from build123d import *

# Parameters (mm, degrees)
SKETCH1_W           = 133.8
SKETCH1_H           = 16.37
SKETCH1_R           = 3.3
BOSS_EXTRUDE1_DEPTH = 1.38
SKETCH2_W           = 1.38
SKETCH2_H           = 16.37
BOSS_EXTRUDE2_DEPTH = 30
FILLET1_R           = 1.5
FILLET2_R           = 0.5
SKETCH3_R           = 2.6
CUT_EXTRUDE1_DEPTH  = 137.56


with BuildPart() as part:
    # Sketch1 → Boss-Extrude1 (new body)
    with BuildSketch(Plane(origin=(0, 0, 0), x_dir=(1, 0, 0), z_dir=(0, 1, 0))):
        with Locations((-5.141278074, 20.650419702)):
            Rectangle(SKETCH1_W, SKETCH1_H)
        with Locations((-30.141278074, 20.650419702)):
            Circle(SKETCH1_R, mode=Mode.SUBTRACT)
        with Locations((19.858721926, 20.650419702)):
            Circle(SKETCH1_R, mode=Mode.SUBTRACT)
    extrude(amount=BOSS_EXTRUDE1_DEPTH)

    # Sketch2 → Boss-Extrude2 (add)
    with BuildSketch(Plane(origin=(0, 1.38, 0), x_dir=(1, 0, 0), z_dir=(0, 1, 0))):
        with Locations((-72.731278074, 20.650419702)):
            Rectangle(SKETCH2_W, SKETCH2_H)
        with Locations((62.448721926, 20.650419702)):
            Rectangle(SKETCH2_W, SKETCH2_H)
    extrude(amount=-BOSS_EXTRUDE2_DEPTH)

    # Fillet1
    fillet1_edges = [part.edges().sort_by_distance(p)[0] for p in [
        (-73.421278074, 1.38, -20.650419702),
        (63.138721926, 1.38, -20.650419702),
    ]]
    fillet(fillet1_edges, radius=FILLET1_R)

    # Fillet2
    fillet2_edges = [part.edges().sort_by_distance(p)[0] for p in [
        (-72.041278074, 0, -20.650419702),
        (61.758721926, 0, -20.650419702),
    ]]
    fillet(fillet2_edges, radius=FILLET2_R)

    # Sketch3 → Cut-Extrude1 (cut, through all)
    with BuildSketch(Plane.ZY.offset(73.421278074)):
        with Locations((-20.650419702, -19.12)):
            Circle(SKETCH3_R)
    extrude(amount=-CUT_EXTRUDE1_DEPTH, mode=Mode.SUBTRACT)


solid = part.part
Input: part model. Units: mm. Frame: model coordinates. A direction names the side the tool comes from. Give positions to 0.01 mm unless a question says otherwise; leave off trailing zeros. Order: outer loops, then holes, each group sorted by start corner. A loop starts at its lowest first (then second) coordinate and runs counter-clockwise, first axis right, second up. Notation, with made-up numbers: (17.25, 3.5) -> (23.25, 3.5) arc R18 ccw to (23.25, 15.5) -> close; hole circle Ø1 at (-28, 83). An arc over 180 degrees is marked (long way). Use one line per item in the form item = value.
1) Section C-C, the plane y = -19.12. Return loops of the section in (x, z).
Response values:
outline = (-73.42, -28.84) -> (-72.04, -28.84) -> (-72.04, -23.25) -> (-73.42, -23.25) -> close; (-73.42, -18.05) -> (-72.04, -18.05) -> (-72.04, -12.47) -> (-73.42, -12.47) -> close; (61.76, -28.84) -> (63.14, -28.84) -> (63.14, -23.25) -> (61.76, -23.25) -> close; (61.76, -18.05) -> (63.14, -18.05) -> (63.14, -12.47) -> (61.76, -12.47) -> close
2) Reachability of faces 5 (the flat face through (61.759, -14, -21)), 6 (the cylindrical face through (19.429, 0.68, -23.922)) from +Z, -Z, +X, -X, +Y, -Y: full face, straight path, thin tool, end or side. Return the list, or none.
Response values:
face_5 = +Z, -Z, -Y
face_6 = +Y, -Y
3) First-contact query: pin 1 Ø5 at (x, z) = (12.5, -21.5) entering from -Y; pin 2 Ø5.5 at (x, z) = (-30.14, -20.65) entering from -Y. Flat tips, straight axial feed; report the tip coordinate or a pass-through.
Response values:
pin_1 = 0
pin_2 = through
4) Line query: probe 1 along X at (y, z) = (-21.25, -27.25); probe 2 along Y at (x, z) = (-52, -14.5). Output: solid intervals per line, ascending.
Response values:
probe_1 = -73.42 to -72.04, 61.76 to 63.14
probe_2 = 0 to 1.38
5) Mould query, pull axis Y, two halves, no side actions, for faces 1 (the cylindrical face through (62.44, -19.01, -23.25)), 2 (the cylindrical face through (-72.74, -19.01, -23.25)), 3 (the flat face through (-6, 1.38, -21)), 4 (the flat face through (-5, 1, -28.835)). Classes: pulls with the +Y half, pulls with the -Y half, needs draft (parallel to the pull), parting line crosses it, or undercut.
Response values:
face_1 = undercut
face_2 = undercut
face_3 = pulls with the +Y half
face_4 = needs draft
6) Section D-D, the plane x = 21. Return loops of the section in (y, z), and give its area (3 significant figures).
Response values:
outline = (0, -28.84) -> (1.38, -28.84) -> (1.38, -23.75) -> (0, -23.75) -> close; (0, -17.55) -> (1.38, -17.55) -> (1.38, -12.47) -> (0, -12.47) -> close
area = 14.0 mm^2
7) Section B-B, the plane z = -25.25. Return loops of the section in (x, y), and give its area (3 significant figures).
Response values:
outline = (-73.42, -28.62) -> (-72.04, -28.62) -> (-72.04, -0.5) arc R0.5 cw to (-71.54, 0) -> (61.26, 0) arc R0.5 cw to (61.76, -0.5) -> (61.76, -28.62) -> (63.14, -28.62) -> (63.14, -0.12) arc R1.5 ccw to (61.64, 1.38) -> (-71.92, 1.38) arc R1.5 ccw to (-73.42, -0.12) -> close
area = 267 mm^2
8) Section A-A, the plane y = -7.5. Return loops of the section in (x, z), and give its area (3 significant figures).
Response values:
outline = (-73.42, -28.84) -> (-72.04, -28.84) -> (-72.04, -12.47) -> (-73.42, -12.47) -> close; (61.76, -28.84) -> (63.14, -28.84) -> (63.14, -12.47) -> (61.76, -12.47) -> close
area = 45.2 mm^2
